Source: CAD feature listing. Evaluate the final solid. Frame: model axes, mm. Face numbers are marked on the shaded views. Round coordinates to 2 decimals unless told otherwise and drop trailing zeros. Loops run counter-clockwise (first coordinate to the right, second up) from the corner with the lowest first, then second, coordinate; pieces in that order, holes last.
Item 1: Section query C-C on y = 4. Return loops of the section in (x, z).
Item 2: Ray query, L1, parallel to Z at x = 0, y = 17; L2, parallel to Y at x = 7.5, z = 4.25; L3, parallel to X at y = 17.25, z = 5. Return the intervals inside material, ascending.
Item 3: Section query A-A on x = 0. Return loops of the section in (y, z), then the cut area to 3 significant figures.
Item 4: Pull-direction query (X, two-part tool) for the marked faces 1, 2 and 3; classes: released by +X, released by -X, zero draft, split by the parting line, or undercut.
Item 5: Section query B-B on z = 8.25. Return loops of the section in (x, y).
Item 6: First-contact query: P1, Ø23, axis at x = 0, y = 0, coming from the +Z side; P2, Ø3.5, axis at x = 0, z = 5, coming from the +Y side; P3, Ø1, axis at x = 14, z = 5.5, coming from the +Y side; P4, Ø3.5, axis at y = 11, z = 7, coming from the -X side. Flat tips, straight axial feed; report the tip coordinate or a pass-through.
Item 7: Section query D-D on x = -4.5. Return loops of the section in (y, z), then the cut area to 3 significant figures.
```python
from build123d import *

# Parameters (mm, degrees)
SKETCH1_R           = 10
BOSS_EXTRUDE1_DEPTH = 10
SKETCH3_W           = 5.5
SKETCH3_H           = 3.5
CUT_EXTRUDE2_DEPTH  = 11
SKETCH4_R           = 2
CUT_EXTRUDE3_DEPTH  = 7


with BuildPart() as part:
    # Sketch1 → Boss-Extrude1 (new body)
    with BuildSketch(Plane.XY):
        with BuildLine():
            Line((-20, 0), (-20, -50))
            Line((-20, -50), (20, -50))
            Line((20, -50), (20, 0))
            ThreePointArc((20, 0), (0, 20), (-20, 0))
        make_face()
        Circle(SKETCH1_R, mode=Mode.SUBTRACT)
    extrude(amount=BOSS_EXTRUDE1_DEPTH)

    # Sketch3 → Cut-Extrude2 (cut)
    with BuildSketch(Plane.XY.offset(10)):
        with Locations((0, 11.25)):
            Rectangle(SKETCH3_W, SKETCH3_H)
    extrude(amount=-CUT_EXTRUDE2_DEPTH, mode=Mode.SUBTRACT)

    # Sketch4 → Cut-Extrude3 (cut)
    with BuildSketch(Plane.XZ.offset(-13)):
        with Locations(Location((0, 5, 0), (0, 0, 270))):
            Circle(SKETCH4_R)
    extrude(amount=-CUT_EXTRUDE3_DEPTH, mode=Mode.SUBTRACT)


solid = part.part
```
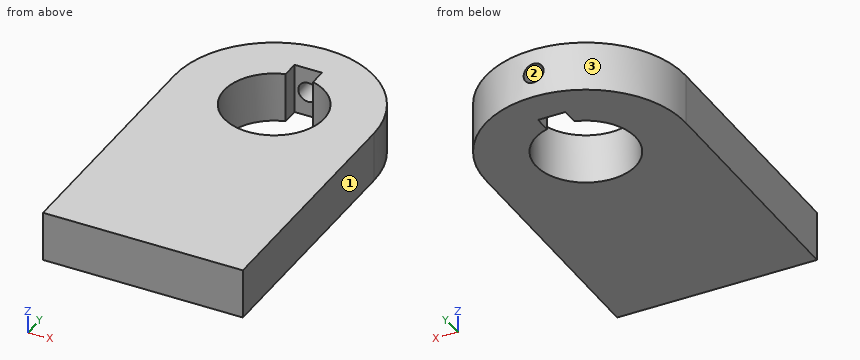
Data:
1. outline: (-19.6, 0) - (-9.17, 0) - (-9.17, 10) - (-19.6, 10) - close; (9.17, 0) - (19.6, 0) - (19.6, 10) - (9.17, 10) - close
2. L1: z = 0 to 3, 7 to 10
2. L2: y = -50 to -6.61, 6.61 to 18.54
2. L3: x = -10.12 to -2, 2 to 10.12
3. outline: (-50, 0) - (-10, 0) - (-10, 10) - (-50, 10) - close; (13, 0) - (20, 0) - (20, 3) - (13, 3) - close; (13, 7) - (20, 7) - (20, 10) - (13, 10) - close
3. area: 442 mm2
4. face 1: released by +X
4. face 2: undercut
4. face 3: split by the parting line
5. outline: (-20, -50) - (20, -50) - (20, 0) arc R20 ccw to (-20, 0) - close; hole (-2.75, 9.61) arc R10 ccw (long way) to (2.75, 9.61) - (2.75, 13) - (-2.75, 13) - close
6. P1: stops at z = 10
6. P2: stops at y = -9.85
6. P3: stops at y = 14.76
6. P4: stops at x = -17.73
7. outline: (-50, 0) - (-8.93, 0) - (-8.93, 10) - (-50, 10) - close; (8.93, 0) - (19.49, 0) - (19.49, 10) - (8.93, 10) - close
7. area: 516 mm2
